from build123d import *

# Parameters (mm, degrees)
F3_DEPTH  = 5
F4_R      = 10
F5_DEPTH  = 2.5
F6_R      = 9
F7_DEPTH  = 10.5
F8_R      = 3
F9_DEPTH  = 12
F10_R     = 3
F11_DEPTH = 18


with BuildPart() as f1:
    # F0 (on Right) → F1 (revolve)
    with BuildSketch(Plane.YZ):
        Polygon((19, 12.5), (0, 12.5), (0, 0), (50, 0), (50, 10), (22, 10), (22, 12.5), (20.5, 12.5), (20.5, 11.5), (19, 11.5), align=None)
    revolve(axis=Axis((0, 25, 0), (0, 1, 0)))

    # F2 (on Front) → F3 (join)
    with BuildSketch(Plane.XZ):
        with BuildLine():
            ThreePointArc((9.4280904158, 11.6666666667), (0, 25), (-9.4280904158, 11.6666666667))
            ThreePointArc((-9.4280904158, 11.6666666667), (-14.9902642074, -0.5403508046), (-8.5636209064, -12.3152099849))
            ThreePointArc((-8.5636209064, -12.3152099849), (-6.8207164782, -14.4547006883), (-6.478218783, -17.1929175614))
            ThreePointArc((-6.478218783, -17.1929175614), (-10.2915186174, -25.9720061348), (-17.9009433962, -31.7780638628))
            ThreePointArc((-17.9009433962, -31.7780638628), (-22.4992996252, -38.7968093702), (-17.7108433735, -45.6872632908))
            ThreePointArc((-17.7108433735, -45.6872632908), (-9.0089982449, -48.1646961023), (0, -49))
            ThreePointArc((0, -49), (9.0089982449, -48.1646961023), (17.7108433735, -45.6872632908))
            ThreePointArc((17.7108433735, -45.6872632908), (22.4992996252, -38.7968093702), (17.9009433962, -31.7780638628))
            ThreePointArc((17.9009433962, -31.7780638628), (10.2915186174, -25.9720061348), (6.478218783, -17.1929175614))
            ThreePointArc((6.478218783, -17.1929175614), (6.8207164782, -14.4547006883), (8.5636209064, -12.3152099849))
            ThreePointArc((8.5636209064, -12.3152099849), (14.9902642074, -0.5403508046), (9.4280904158, 11.6666666667))
        make_face()
    extrude(amount=F3_DEPTH)

    # F4 (on face) → F5 (join)
    with BuildSketch(Plane.XZ.offset(5)):
        with Locations((0, 15)):
            Circle(F4_R)
    extrude(amount=F5_DEPTH)

    # F6 (on face) → F7 (join)
    with BuildSketch(Plane.XZ.offset(7.5)):
        with Locations((0, 15)):
            Circle(F6_R)
    extrude(amount=F7_DEPTH)

    # F8 (on face) → F9 (cut)
    with BuildSketch(Plane.XZ.offset(18)):
        with Locations((0, 15)):
            Circle(F8_R)
    extrude(amount=-F9_DEPTH, mode=Mode.SUBTRACT)

    # F10 (on face) → F11 (cut)
    with BuildSketch(Plane(origin=(0, 50, 0), x_dir=(-1, 0, 0), z_dir=(0, 1, 0))):
        Circle(F10_R)
    extrude(amount=-F11_DEPTH, mode=Mode.SUBTRACT)


solid = f1.part
Work out the finished part from the listing and answer in its coordinate system (mm). A direction names the side the tool comes from. Give positions to 0.01 mm unless a question says otherwise; leave off trailing zeros. Loops run counter-clockwise (first coordinate to the right, second up) from the corner with the lowest first, then second, coordinate; pieces in that order, holes last. Notation, with made-up numbers: (83.5, 42) -> (130.5, 42) arc R24 cw to (130.5, 80) -> close; hole circle Ø3 at (54.5, 48). An arc over 180 degrees is marked (long way). Use a Markdown table: item, result. Add a question column.
1) The part is cut by section C-C, the plane y = 4. Determine the outline of the cut face in (x, z).
2) The part is cut by section B-B, the plane y = 46.5. Determine the outline of the cut face in (x, z), plus the area to 3 significant figures.
3) The part is cut by section D-D, the plane x = -5.5. Determine the outline of the cut face in (y, z), plus the area to 3 significant figures.
4) Which of the six approach directions +Z, -Z, +X, -X, +Y, -Y give full straight-line access (tool end or side, diameter ignored) to faces 1 (the flat face through (-9, -7.5, 17)), 2 (the cylindrical face through (11.4, 19.7, -1.5)), 3 (the cylindrical face through (10.375, -2.465, -26.078)), 4 (the flat face through (10.2, 22, 0.1))?
5) For a pull along Z with two mould halves and no side action, classify faces 5 (the flat face through (-4, 19, -11)), 6 (the flat face through (0, 32, 0)), 7 (the cylindrical face through (3.755, 9.367, 11.923)) as +Z half, -Z half, draft (parallel to the pull), parting line (faces both ways), or undercut.
6) Each of these flat-tipped pins is pushed along its axis until it touches: P1, Ø5, axis at x = -10.5, y = -2, coming from the +Z side; P2, Ø13.5, axis at x = 8.5, z = -26.5, coming from the -Y side; P3, Ø5, axis at x = -12.5, z = -14.5, coming from the -Y side; P4, Ø4, axis at y = -2.5, z = -5, coming from the +X side. Where does it stop, or does it pass through?
7) Consider line 1 along Y through (x, z) = (7, -9.5); line 2 along Z through (x, y) = (0, -13.25); line 3 along Y through (x, z) = (-9, -29). Determine where each line is inside the solid, lowest interval first.
8) The part is cut by section A-A, the plane z = 0. Determine the outline of the cut face in (x, y).
Reported:
| question | item | result |
|---|---|---|
| 1 | outline | circle Ø25 at (0, 0) |
| 2 | outline | circle Ø20 at (0, 0); hole circle Ø6 at (0, 0) |
| 2 | area | 286 mm^2 |
| 3 | outline | (-18, 7.88) -> (-7.5, 7.88) -> (-7.5, 6.65) -> (-5, 6.65) -> (-5, -48.69) -> (0, -48.69) -> (0, -11.22) -> (19, -11.22) -> (19, -10.1) -> (20.5, -10.1) -> (20.5, -11.22) -> (22, -11.22) -> (22, -8.35) -> (50, -8.35) -> (50, 8.35) -> (22, 8.35) -> (22, 11.22) -> (20.5, 11.22) -> (20.5, 10.1) -> (19, 10.1) -> (19, 11.22) -> (0, 11.22) -> (0, 23.35) -> (-7.5, 23.35) -> (-7.5, 22.12) -> (-18, 22.12) -> close |
| 3 | area | 1,510 mm^2 |
| 4 | face 1 | -Y |
| 4 | face 2 | none |
| 4 | face 3 | +X, +Y, -Y |
| 4 | face 4 | +Y |
| 5 | face 5 | draft |
| 5 | face 6 | undercut |
| 5 | face 7 | parting line |
| 6 | P1 | stops at z = 21 |
| 6 | P2 | stops at y = -5 |
| 6 | P3 | passes through |
| 6 | P4 | stops at x = 14.7 |
| 7 | line 1 | y = -5 to 19, 20.5 to 22 |
| 7 | line 2 | z = 6 to 12, 18 to 24 |
| 7 | line 3 | y = -5 to 0 |
| 8 | outline | (-15, -5) -> (15, -5) -> (15, 0) -> (12.5, 0) -> (12.5, 19) -> (11.5, 19) -> (11.5, 20.5) -> (12.5, 20.5) -> (12.5, 22) -> (10, 22) -> (10, 50) -> (3, 50) -> (3, 32) -> (-3, 32) -> (-3, 50) -> (-10, 50) -> (-10, 22) -> (-12.5, 22) -> (-12.5, 20.5) -> (-11.5, 20.5) -> (-11.5, 19) -> (-12.5, 19) -> (-12.5, 0) -> (-15, 0) -> close |
